Work out the finished part from the listing and answer in its coordinate system (mm). A direction names the side the tool comes from. Give positions to 0.01 mm unless a question says otherwise; leave off trailing zeros. Order: outer loops, then holes, each group sorted by start corner. A loop starts at its lowest first (then second) coordinate and runs counter-clockwise, first axis right, second up.
```python
from build123d import *

# Parameters (mm, degrees)
F1_R     = 8.89
F1_R_2   = 5.969
F3_DEPTH = 3.556
F5_R     = 8.89
F5_R_2   = 7.62
F7_DEPTH = 3.556


# Not quite as in the source:
# - a feature of the source that left no trace in its solid (it failed there, or was rolled back) is left out
# - a pattern or mirror of a feature is missing from the dataset's text; its kind, count and spacing are read off the source's solid


with BuildPart() as f2:
    # F2: sweep along a path in F0
    with BuildLine(Plane.XY) as f2_path:
        Line((0, 0), (0, 9.7015046))
        ThreePointArc((0, 9.7015046), (13.97, 23.6715046), (27.94, 9.7015046))
        Line((27.94, 9.7015046), (27.94, 0))
        Line((27.94, 0), (27.94, -3.556))
    # F1 (on Front) → F2 (sweep)
    with BuildSketch(Plane.XZ):
        Circle(F1_R)
        Circle(F1_R_2, mode=Mode.SUBTRACT)
    sweep(path=f2_path.line)

    # F3 (add): a face of the model
    f3_faces = [f2.faces().sort_by_distance(p)[0] for p in [
        (-8.6385528286, 0, 0),
    ]]
    extrude(f3_faces, amount=F3_DEPTH)

    # F5 (on face) → F7 (cut)
    with BuildSketch(Plane.XZ.offset(3.556)):
        with Locations((27.94, 0)):
            Circle(F5_R)
        with Locations((27.94, 0)):
            Circle(F5_R_2, mode=Mode.SUBTRACT)
    f7 = extrude(amount=-F7_DEPTH, mode=Mode.SUBTRACT)

    # F7_copies: F7 across plane
    add(f7.mirror(Plane(origin=(13.97, 0, 0), x_dir=(0, 0, -1), z_dir=(-1, 0, 0))), mode=Mode.SUBTRACT)


solid = f2.part
```
1. Given P1, Ø5.5, axis at x = -3.5, z = 2.5, coming from the -Y side; P2, Ø6, axis at x = 16.5, z = -2.5, coming from the +Y side; P3, Ø7, axis at x = 27.94, z = 0, coming from the +Y side; P4, Ø4, axis at y = 4, z = -3, coming from the +X side, each flat-ended and moving along its own axis, determine where each tip first touches the part or whether it passes through.
Findings below:
P1: stops at y = -3.56
P2: stops at y = 32.55
P3: stops at y = 30.02
P4: stops at x = 36.77
2. The part is cut by section C-C (z = 3.5). Write down the section's boundary in (x, y), then the cut area to 3 significant figures.
Findings below:
outline: (-8.17, 0) - (-6.77, 0) - (-6.77, -3.56) - (-4.84, -3.56) - (-4.84, 9.7) arc R18.81 cw to (32.78, 9.7) - (32.78, -3.56) - (34.71, -3.56) - (34.71, 0) - (36.11, 0) - (36.11, 9.7) arc R22.14 ccw to (-8.17, 9.7) - close; (4.84, -3.56) - (6.77, -3.56) - (6.77, 0) - (8.17, 0) - (8.17, 9.7) arc R5.8 cw to (19.77, 9.7) - (19.77, 0) - (21.17, 0) - (21.17, -3.56) - (23.1, -3.56) - (23.1, 9.7) arc R9.13 ccw to (4.84, 9.7) - close
area: 450 mm2
3. Which of the six approach directions +Z, -Z, +X, -X, +Y, -Y give full straight-line access (tool end or side, diameter ignored) to faces 4 (the face through (35.208, -1.803, 2.289)), 5 (the face through (24, -3.556, -5))?
Findings below:
face 4: -Y
face 5: +Z, -Z, +X, -X, -Y
4. The part is cut by section A-A (y = -1). Write down the section's boundary in (x, z).
Findings below:
outline: circle Ø15.24 at (0, 0); circle Ø15.24 at (27.94, 0); hole circle Ø11.94 at (0, 0); hole circle Ø11.94 at (27.94, 0)
5. The mould has two halves that part along Z. Classify faces 1 (the face through (-7, 0, 4)), 2 (the face through (-1.93, 4.92, 8.68)), 3 (the face through (33.9, 3, -0.3)): pulls with the +Z half, pulls with the -Z half, needs draft (parallel to the pull), parting line crosses it, or undercut.
Findings below:
face 1: needs draft
face 2: parting line crosses it
face 3: undercut
6. Straight lines are drawn through the part: probe 1 along X at (y, z) = (3.5, 0); probe 2 along X at (y, z) = (1, 2.75); probe 3 along Z at (x, y) = (27.94, 1.25). For each, find the intervals that lie inside material, in ascending order.
Findings below:
probe 1: x = -8.89 to -5.97, 5.97 to 8.89, 19.05 to 21.97, 33.91 to 36.83
probe 2: x = -8.45 to -5.3, 5.3 to 8.45, 19.49 to 22.64, 33.24 to 36.39
probe 3: z = -8.89 to -5.97, 5.97 to 8.89
7. The part is cut by section D-D (y = 7). Write down the section's boundary in (x, z), then the cut area to 3 significant figures.
Findings below:
outline: circle Ø17.78 at (0, 0); circle Ø17.78 at (27.94, 0); hole circle Ø11.94 at (0, 0); hole circle Ø11.94 at (27.94, 0)
area: 273 mm2
8. The part is cut by section B-B (z = 0). Write down the section's boundary in (x, y), then the cut area to 3 significant figures.
Findings below:
outline: (-8.89, 0) - (-7.62, 0) - (-7.62, -3.56) - (-5.97, -3.56) - (-5.97, 9.7) arc R19.94 cw to (33.91, 9.7) - (33.91, -3.56) - (35.56, -3.56) - (35.56, 0) - (36.83, 0) - (36.83, 9.7) arc R22.86 ccw to (-8.89, 9.7) - close; (5.97, -3.56) - (7.62, -3.56) - (7.62, 0) - (8.89, 0) - (8.89, 9.7) arc R5.08 cw to (19.05, 9.7) - (19.05, 0) - (20.32, 0) - (20.32, -3.56) - (21.97, -3.56) - (21.97, 9.7) arc R8 ccw to (5.97, 9.7) - close
area: 393 mm2
